Part model, mm, in its own coordinate system. Face numbers are marked on the shaded views. A direction names the side the tool comes from. Give positions to 0.01 mm unless a question says otherwise; leave off trailing zeros. Order: outer loops, then holes, each group sorted by start corner. A loop starts at its lowest first (then second) coordinate and runs counter-clockwise, first axis right, second up.
1. Drop a flat-ended pin along its axis: pin 1 Ø2 at (x, y) = (-1.5, 7) entering from -Z. Give the stop position or say it passes through.
2. Probe line 1 (Y direction, x = -1.4, z = 0.5); line 2 (X direction, y = 4.25, z = -0.1); line 3 (Y direction, x = -0.5, z = -0.05). List the from-to ranges inside material, lowest first.
3. Which spindle directions (+Z, -Z, +X, -X, +Y, -Y) get a long thin tool onto all of the face, cutting with end or side? Do the marked faces 1, 2 and 3. Say none if no direction does.
4. Slice it at C-C on x = -1.5. List the corners of the cut face in (y, z).
5. Slice it at A-A on x = 0. List the corners of the cut face in (y, z), and give its area (3 significant figures).
6. Slice it at B-B on y = 7.5. List the corners of the cut face in (x, z), and give its area (3 significant figures).
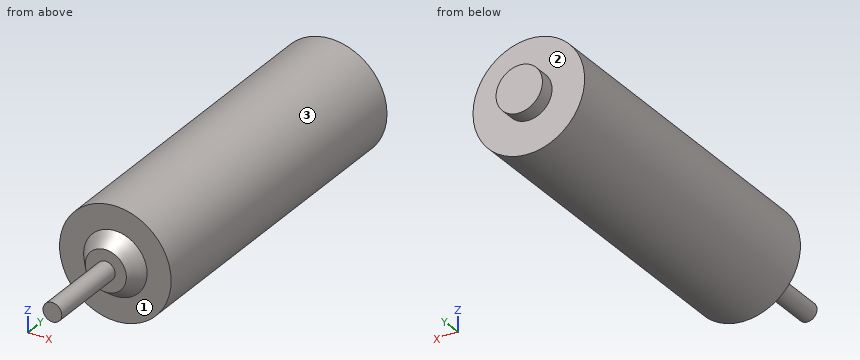
from build123d import *

# Parameters (mm, degrees)
F0_R     = 2.032
F1_DEPTH = 12.319
F2_R     = 0.84455
F3_DEPTH = 0.5461
F4_R     = 1.1557
F6_R     = 0.7493
F8_R     = 0.3429
F9_DEPTH = 3.048


with BuildPart() as f1:
    # F0 (on Front) → F1 (new body)
    with BuildSketch(Plane.XZ):
        Circle(F0_R)
    extrude(amount=-F1_DEPTH)

    # F2 (on face) → F3 (join)
    with BuildSketch(Plane(origin=(0, 12.319, 0), x_dir=(-1, 0, 0), z_dir=(0, 1, 0))):
        Circle(F2_R)
    extrude(amount=F3_DEPTH)

    # F4 (on face) → F7 section 0
    with BuildSketch(Plane.XZ):
        Circle(F4_R)
    # F6 (on offset) → F7 section 1
    with BuildSketch(Plane.XZ.offset(0.5461)):
        Circle(F6_R)
    loft()

    # F8 (on face) → F9 (join)
    with BuildSketch(Plane.XZ.offset(0.5461)):
        Circle(F8_R)
    extrude(amount=F9_DEPTH)


solid = f1.part
Data:
1. pin 1: stops at z = -1.97
2. line 1: y = 0 to 12.32
2. line 2: x = -2.03 to 2.03
2. line 3: y = -0.55 to 12.87
3. face 1: -Y
3. face 2: +Y
3. face 3: +Y, -Y
4. outline: (0, -1.37) - (12.32, -1.37) - (12.32, 1.37) - (0, 1.37) - close
5. outline: (-3.59, -0.34) - (-0.55, -0.34) - (-0.55, -0.75) - (0, -1.16) - (0, -2.03) - (12.32, -2.03) - (12.32, -0.84) - (12.87, -0.84) - (12.87, 0.84) - (12.32, 0.84) - (12.32, 2.03) - (0, 2.03) - (0, 1.16) - (-0.55, 0.75) - (-0.55, 0.34) - (-3.59, 0.34) - close
5. area: 54.1 mm2
6. outline: circle Ø4.06 at (0, 0)
6. area: 13.0 mm2
